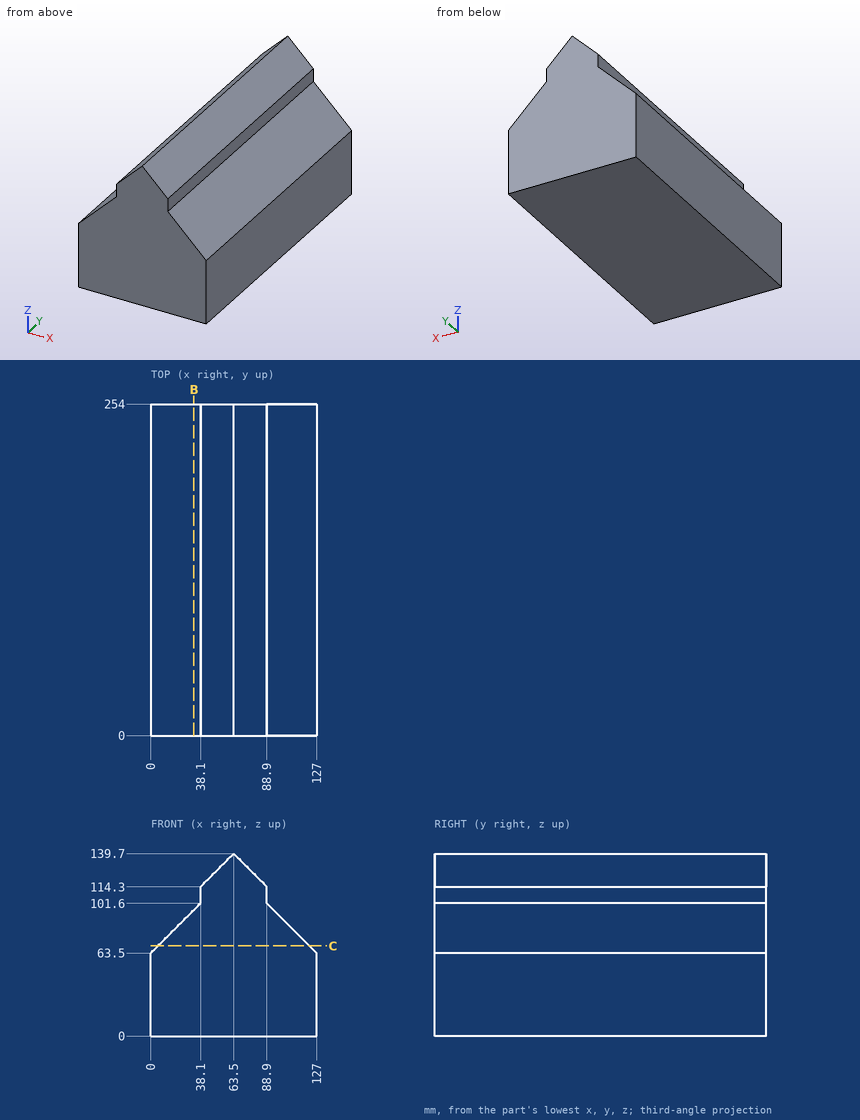
Drawing for the job (mm, zero at the part's lowest x, y, z). Give positions to 0.01 mm unless a question says otherwise; leave off trailing zeros. Loops run counter-clockwise (first coordinate to the right, second up) from the corner with the lowest first, then second, coordinate; pieces in that order, holes last.
Item 1: Drop flat-ended pins along their axis: P1, Ø14, axis at y = 162.5, z = 111, coming from the -X side; P2, Ø10, axis at y = 189.5, z = 108.5, coming from the +X side; P3, Ø5, axis at y = 204.5, z = 99.5, coming from the -X side. Give the stop position or say it passes through.
Check values:
P1: stops at x = 38.1
P2: stops at x = 88.9
P3: stops at x = 33.5
Item 2: Drill centre lines: line 1 along Z through (x, y) = (89, 37.5); line 2 along X through (y, z) = (98, 96); line 3 along X through (y, z) = (49.5, 93.5). Where is each one in solid material? Low to high.
Check values:
line 1: z = 0 to 101.5
line 2: x = 32.5 to 94.5
line 3: x = 30 to 97
Item 3: Slice it at C-C (z = 69). Write the cut outline in (x, y).
Check values:
outline: (5.5, 0) - (121.5, 0) - (121.5, 254) - (5.5, 254) - close
Item 4: Slice it at B-B (x = 33). Write the cut outline in (y, z), plus the area to 3 significant figures.
Check values:
outline: (0, 0) - (254, 0) - (254, 96.5) - (0, 96.5) - close
area: 24,500 mm2
